Source: three-view drawing plus pictorial views. Frame: mm from the lowest corner of the part. A direction names the side the tool comes from. Give positions to 0.01 mm unless a question says otherwise; leave off trailing zeros. Order: outer loops, then holes, each group sorted by start corner. A loop starts at its lowest first (then second) coordinate and runs counter-clockwise, first axis right, second up.
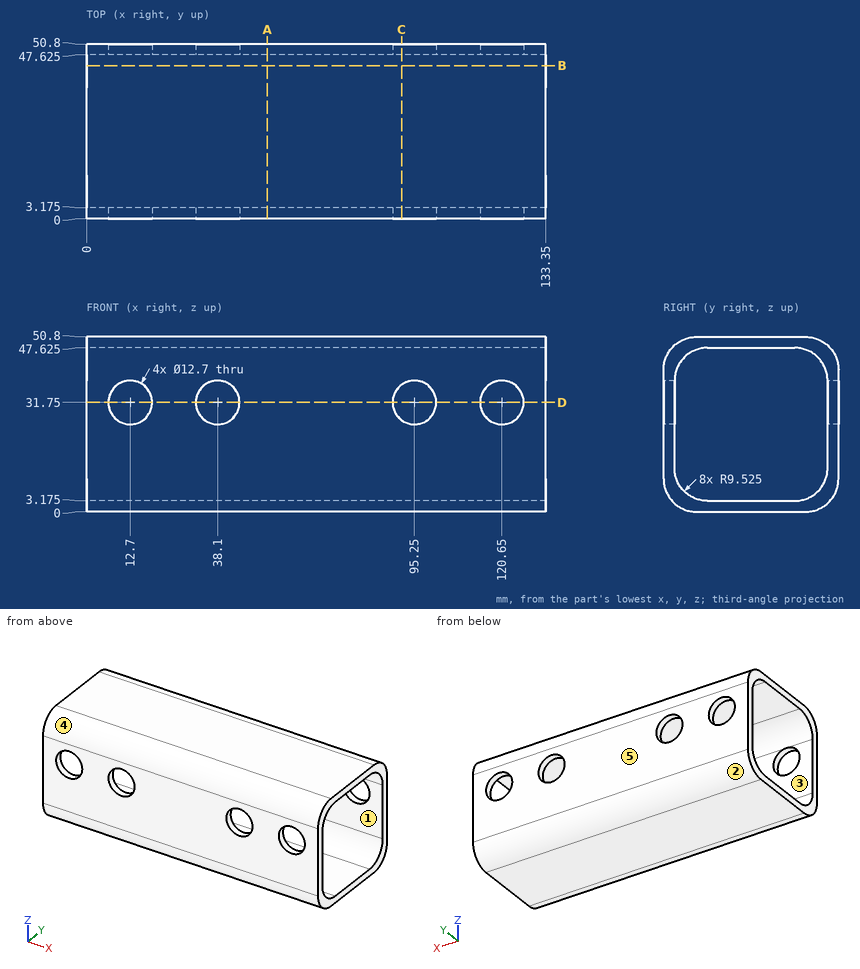
1) Section query C-C on x = 91.5. Output: boundary loops of the cut face in (y, z) (3 decimals), and give its area (3 significant figures).
Checks:
outline: (0, 9.525) arc R9.525 ccw to (9.525, 0) - (41.275, 0) arc R9.525 ccw to (50.8, 9.525) - (50.8, 26.626) - (47.625, 26.626) - (47.625, 12.7) arc R9.525 cw to (38.1, 3.175) - (12.7, 3.175) arc R9.525 cw to (3.175, 12.7) - (3.175, 26.626) - (0, 26.626) - close; (0, 36.874) - (3.175, 36.874) - (3.175, 38.1) arc R9.525 cw to (12.7, 47.625) - (38.1, 47.625) arc R9.525 cw to (47.625, 38.1) - (47.625, 36.874) - (50.8, 36.874) - (50.8, 41.275) arc R9.525 ccw to (41.275, 50.8) - (9.525, 50.8) arc R9.525 ccw to (0, 41.275) - close
area: 540 mm2
2) Section query B-B on y = 44.5. Output: boundary loops of the cut face in (x, z).
Checks:
outline: (0, 0.56) - (133.35, 0.56) - (133.35, 5.65) - (0, 5.65) - close; (0, 45.15) - (133.35, 45.15) - (133.35, 50.24) - (0, 50.24) - close
3) Pull-direction query (Z, two-part tool) for the marked faces 3, 4 and 5; classes: +Z half, -Z half, draft (parallel to the pull), parting line (faces both ways), or undercut.
Checks:
face 3: undercut
face 4: +Z half
face 5: draft
4) Ray query, L1, parallel to X at y = 48.35, z = 31.75; L2, parallel to Z at x = 73.5, y = 16 (3 decimals). Return the intervals inside material, ascending.
Checks:
L1: x = 0 to 6.35, 19.05 to 31.75, 44.45 to 88.9, 101.6 to 114.3, 127 to 133.35
L2: z = 0 to 3.175, 47.625 to 50.8
5) Reachability of the marked faces 1 and 2 from +Z, -Z, +X, -X, +Y, -Y: full face, straight path, thin tool, end or side. Return the list, or none.
Checks:
face 1: +X, -X
face 2: -Z, +X, -X, +Y
6) Section query D-D on z = 31.75. State how many separate pieces and enclosed holes the cut face has, and give its area (3 significant figures).
Checks:
separate pieces: 10
enclosed holes: 0
area: 524 mm2
7) Section query A-A on x = 52.5. Output: boundary loops of the cut face in (y, z) (3 decimals), and give its area (3 significant figures).
Checks:
outline: (0, 9.525) arc R9.525 ccw to (9.525, 0) - (41.275, 0) arc R9.525 ccw to (50.8, 9.525) - (50.8, 41.275) arc R9.525 ccw to (41.275, 50.8) - (9.525, 50.8) arc R9.525 ccw to (0, 41.275) - close; hole (3.175, 12.7) arc R9.525 ccw to (12.7, 3.175) - (38.1, 3.175) arc R9.525 ccw to (47.625, 12.7) - (47.625, 38.1) arc R9.525 ccw to (38.1, 47.625) - (12.7, 47.625) arc R9.525 ccw to (3.175, 38.1) - close
area: 605 mm2
8) First-contact query: pin 1 Ø7.5 at (x, z) = (38.1, 31.75) entering from -Y. Flat tip, straight axial feed; report the tip coordinate or a pass-through.
Checks:
pin 1: passes through
